Model file for the job. Use its own axes, mm. A direction names the side the tool comes from. Coordinates: 2 decimals unless noted, no trailing zeros. Loops run counter-clockwise (first coordinate to the right, second up) from the corner with the lowest first, then second, coordinate; pieces in that order, holes last. Notation, with made-up numbers: M 56,33 L 107,33 A20 ccw 107,67 Z; hole C 2.25,-31 d6. An arc over 180 degrees is marked long. One line per question, with ' | ' between items. Start each with the question number.
```python
from build123d import *

# Parameters (mm, degrees)
SKETCH1_R           = 30
BOSS_EXTRUDE1_DEPTH = 40
CUT_EXTRUDE1_START  = -5
SKETCH2_OUTSIDE_W   = 80.762
SKETCH2_OUTSIDE_H   = 80.762
SKETCH2_OUTSIDE_R   = 17.5
CUT_EXTRUDE1_DEPTH  = 30
SKETCH3_R           = 2
CUT_EXTRUDE2_DEPTH  = 59.309518948
CUT_EXTRUDE3_DEPTH  = 59.309518948
CUT_EXTRUDE4_REACH  = 57
SKETCH5_R           = 2


with BuildPart() as part:
    # Sketch1 → Boss-Extrude1 (new body)
    with BuildSketch(Plane(origin=(0, 0, 0), x_dir=(1, 0, 0), z_dir=(0, 1, 0))):
        with Locations(Location((0, 0, 0), (0, 0, 270))):
            Circle(SKETCH1_R)
    extrude(amount=BOSS_EXTRUDE1_DEPTH)

    # Sketch2 outside → Cut-Extrude1 (cut)
    with BuildSketch(Plane.XZ.offset(CUT_EXTRUDE1_START)):
        Rectangle(SKETCH2_OUTSIDE_W, SKETCH2_OUTSIDE_H)
        with Locations(Location((0, 0, 0), (0, 0, 270))):
            Circle(SKETCH2_OUTSIDE_R, mode=Mode.SUBTRACT)
    extrude(amount=-CUT_EXTRUDE1_DEPTH, mode=Mode.SUBTRACT)

    # Sketch3 → Cut-Extrude2 (cut, through all)
    with BuildSketch(Plane.XZ):
        with Locations(Location((0, 0, 0), (0, 0, 270))):
            Circle(SKETCH3_R)
    extrude(amount=-CUT_EXTRUDE2_DEPTH, mode=Mode.SUBTRACT)

    # Sketch4 → Cut-Extrude3 (cut, through all)
    with BuildSketch(Plane.XZ):
        with BuildLine():
            ThreePointArc((5.314601624, -8.562564428), (0.136244015, -3.747524192), (-4.678796221, -8.925881801))
            Line((-4.678796221, -8.925881801), (5.314601624, -8.562564428))
        make_face()
        with BuildLine():
            Line((5.314601624, -8.562564428), (-4.678796221, -8.925881801))
            ThreePointArc((-4.678796221, -8.925881801), (0.40874704, -13.743397777), (5.317902702, -8.744223114))
            ThreePointArc((5.317902702, -8.744223114), (5.317077364, -8.653378776), (5.314601624, -8.562564428))
        make_face()
        with BuildLine():
            ThreePointArc((4.758097504, 8.883862231), (3.177329144, 1.991752874), (10.069438501, 0.410984514))
            Line((10.069438501, 0.410984514), (4.758097504, 8.883862231))
        make_face()
        with BuildLine():
            Line((4.758097504, 8.883862231), (10.069438501, 0.410984514))
            ThreePointArc((10.069438501, 0.410984514), (11.788602428, 2.226509547), (12.413768003, 4.647423373))
            ThreePointArc((12.413768003, 4.647423373), (9.834681829, 9.022257798), (4.758097504, 8.883862231))
        make_face()
        with BuildLine():
            ThreePointArc((-5.39064228, 8.514897287), (-12.149768249, 6.437828165), (-10.072699128, -0.321297804))
            Line((-10.072699128, -0.321297804), (-5.39064228, 8.514897287))
        make_face()
        with BuildLine():
            Line((-5.39064228, 8.514897287), (-10.072699128, -0.321297804))
            ThreePointArc((-10.072699128, -0.321297804), (-5.153409868, -0.187190345), (-2.731670704, 4.096799742))
            ThreePointArc((-2.731670704, 4.096799742), (-3.447680618, 6.675060578), (-5.39064228, 8.514897287))
        make_face()
    extrude(amount=-CUT_EXTRUDE3_DEPTH, mode=Mode.SUBTRACT)

    # Sketch5 → Cut-Extrude4 (cut, up to next)
    with BuildSketch(Plane(origin=(0, 5, 0), x_dir=(1, 0, 0), z_dir=(0, 1, 0)), mode=Mode.PRIVATE) as cut_extrude4_sk1:
        with Locations(Location((-15.339737127, 8.422734999, 0), (0, 0, 270))):
            Circle(SKETCH5_R)
    cut_extrude4_tool1 = extrude(cut_extrude4_sk1.sketch, amount=-CUT_EXTRUDE4_REACH, mode=Mode.PRIVATE) & part.part
    add(cut_extrude4_tool1.solids().sort_by_distance((-15.339737, 5, -8.422735))[0], mode=Mode.SUBTRACT)


solid = part.part
```
(1) 3-axis set-ups, long thin cutter, end or side, ignore diameter. For faces 1 (the face through (0, 0, 6)), 2 (the face through (13, 35, -13)), 3 (the face through (-14, 5, -8)): which of +Z, -Z, +X, -X, +Y, -Y reach the whole face in a straight line?
(2) Band-saw the part on D-D on y = 36. Write the cut outline in (x, z).
(3) Two-plate mould, pull along Z, no slides. Class faces 4 (the face through (0, 40, 6)), 5 (the face through (-10.648, 19.79, 13.887)), 6 (the face through (-16.557, 2.535, -10.01)): pulls with the +Z half, pulls with the -Z half, needs draft (parallel to the pull), parting line crosses it, or undercut.
(4) Drill centre lines: line 1 (Y direction, x = 20.5, z = 2.5); line 2 (Z direction, x = 8, y = 30); line 3 (X direction, y = 35.5, z = -8.5). Where is each one in solid material? Low to high. Write a range as [from, to].
(5) Band-saw the part on A-A on y = 17. Write the cut outline in (x, z), then the cut area to 3 significant figures.
(6) Band-saw the part on B-B on z = -22. Write the cut outline in (x, y).
(7) Pin check, flat tips, straight feed: P1, Ø3.5, axis at x = -15.34, z = -8.42, coming from the -Y side; P2, Ø12, axis at x = 3, z = 1, coming from the -Y side; P3, Ø4, axis at y = 16, z = -15.5, coming from the -X side; P4, Ø1, axis at x = 8.5, y = 7, coming from the -Z side. Stop position of each tip, or through.
(8) Band-saw the part on C-C on x = 0. Write the cut outline in (y, z), then the cut area to 3 significant figures.
Computed values:
1) face 1: +Z, -Z, +X, -X, -Y | face 2: none | face 3: -Y
2) outline: C 0,0 d60; hole C -7.73,4.1 d10; hole C 0,0 d4; hole C 7.41,4.65 d10; hole M 5.31,-8.56 A5 ccw long 5.32,-8.74 A5 ccw Z
3) face 4: needs draft | face 5: parting line crosses it | face 6: undercut
4) line 1: [0, 5], [35, 40] | line 2: [-15.56, -0.32], [9.61, 15.56] | line 3: [-28.77, -4.68], [5.31, 28.77]
5) outline: C 0,0 d35; hole C -7.73,4.1 d10; hole C 0,0 d4; hole C 7.41,4.65 d10; hole M 5.31,-8.56 A5 ccw long 5.32,-8.74 A5 ccw Z | area: 714 mm^2
6) outline: M -20.4,0 L 20.4,0 L 20.4,5 L -20.4,5 Z; M -20.4,35 L 20.4,35 L 20.4,40 L -20.4,40 Z
7) P1: y = 5 | P2: y = 0 | P3: x = -11.14 | P4: z = -15.56
8) outline: M 0,-30 L 5,-30 L 5,-17.5 L 35,-17.5 L 35,-30 L 40,-30 L 40,-13.73 L 0,-13.73 Z; M 0,-3.75 L 40,-3.75 L 40,-2 L 0,-2 Z; M 0,2 L 40,2 L 40,30 L 35,30 L 35,17.5 L 5,17.5 L 5,30 L 0,30 Z | area: 1,090 mm^2
